Check sheet for the modelled part. Datum: model origin and axes. Units: mm. Face numbers are marked on the shaded views. A direction names the side the tool comes from. Round coordinates to 2 decimals unless told otherwise and drop trailing zeros. Loops run counter-clockwise (first coordinate to the right, second up) from the corner with the lowest first, then second, coordinate; pieces in that order, holes last. Notation, with made-up numbers: (-2.5, 48.25) - (42.5, 48.25) arc R19 cw to (42.5, 82.25) - close; hole circle Ø10 at (-5, 74.5). An arc over 180 degrees is marked (long way). Return JSON: item names as keys, results as strings.
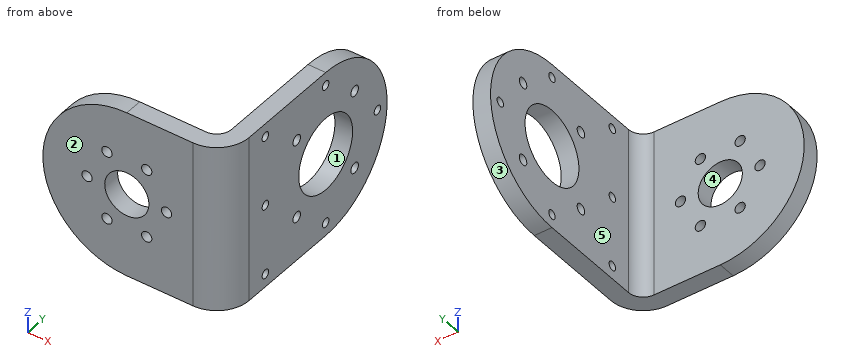
from build123d import *

# Parameters (mm, degrees)
EXTRUDE_1_DEPTH     = 6
EXTRUDE_2_DEPTH     = 6
SKETCH_4_R          = 1.75
CUT_EXTRUDE_1_DEPTH = 16
SKETCH_6_R          = 1.75
CUT_EXTRUDE_2_DEPTH = 16
FILLET_1_R          = 5
FILLET_2_R          = 11
SKETCH_7_R          = 1.5
SKETCH_7_R_2        = 12.5
CUT_EXTRUDE_3_DEPTH = 10
SKETCH_8_R          = 7.5
CUT_EXTRUDE_4_DEPTH = 10


with BuildPart() as part:
    # 草图1 → 凸台-拉伸1 (new body)
    with BuildSketch(Plane(origin=(0, 0, 0), x_dir=(1, 0, 0), z_dir=(0, 1, 0))):
        with BuildLine():
            ThreePointArc((0, 28.5), (-28.5, 0), (0, -28.5))
            Line((0, -28.5), (33.5, -28.5))
            Line((33.5, -28.5), (33.5, 28.5))
            Line((33.5, 28.5), (0, 28.5))
        make_face()
    extrude(amount=EXTRUDE_1_DEPTH)

    # 草图3 → 凸台-拉伸2 (add)
    with BuildSketch(Plane(origin=(33.5, 0, 0), x_dir=(0, 0, -1), z_dir=(1, 0, 0))):
        with BuildLine():
            Line((-28.5, 46.5), (-28.5, 6))
            Line((-28.5, 6), (28.5, 6))
            Line((28.5, 6), (28.5, 46.5))
            ThreePointArc((28.5, 46.5), (0, 75), (-28.5, 46.5))
        make_face()
    extrude(amount=-EXTRUDE_2_DEPTH)

    # 草图4 → 切除-拉伸1 (cut)
    with BuildSketch(Plane(origin=(0, 6, 0), x_dir=(1, 0, 0), z_dir=(0, 1, 0))):
        with Locations(Location((-13.5, 0, 0), (0, 0, 270))):
            Circle(SKETCH_4_R)
        with Locations(Location((-6.75, 11.691342951, 0), (0, 0, 270))):
            Circle(SKETCH_4_R)
        with Locations(Location((6.75, 11.691342951, 0), (0, 0, 270))):
            Circle(SKETCH_4_R)
        with Locations(Location((13.5, 0, 0), (0, 0, 270))):
            Circle(SKETCH_4_R)
        with Locations(Location((6.75, -11.691342951, 0), (0, 0, 270))):
            Circle(SKETCH_4_R)
        with Locations(Location((-6.75, -11.691342951, 0), (0, 0, 270))):
            Circle(SKETCH_4_R)
    extrude(amount=-CUT_EXTRUDE_1_DEPTH, mode=Mode.SUBTRACT)

    # 草图6 → 切除-拉伸2 (cut)
    with BuildSketch(Plane(origin=(33.5, 0, 0), x_dir=(0, 0, -1), z_dir=(1, 0, 0))):
        with Locations((-13.435028843, 59.935028843)):
            Circle(SKETCH_6_R)
        with Locations((13.435028843, 59.935028843)):
            Circle(SKETCH_6_R)
        with Locations((13.435028843, 33.064971157)):
            Circle(SKETCH_6_R)
        with Locations((-13.435028843, 33.064971157)):
            Circle(SKETCH_6_R)
    extrude(amount=-CUT_EXTRUDE_2_DEPTH, mode=Mode.SUBTRACT)

    # 圆角1
    fillet_1_edges = [part.edges().sort_by_distance(p)[0] for p in [
        (27.5, 6, 0),
    ]]
    fillet(fillet_1_edges, radius=FILLET_1_R)

    # 圆角2
    fillet_2_edges = [part.edges().sort_by_distance(p)[0] for p in [
        (33.5, 0, 0),
    ]]
    fillet(fillet_2_edges, radius=FILLET_2_R)

    # 草图7 → 切除-拉伸3 (cut)
    with BuildSketch(Plane(origin=(33.5, 0, 0), x_dir=(0, 0, -1), z_dir=(1, 0, 0))):
        with Locations((0, 70.5)):
            Circle(SKETCH_7_R)
        with Locations((-24, 46.5)):
            Circle(SKETCH_7_R)
        with Locations((24, 46.5)):
            Circle(SKETCH_7_R)
        with Locations((-24, 18.5)):
            Circle(SKETCH_7_R)
        with Locations((24, 18.5)):
            Circle(SKETCH_7_R)
        with Locations((0, 18.5)):
            Circle(SKETCH_7_R)
        with Locations((0, 46.5)):
            Circle(SKETCH_7_R_2)
    extrude(amount=-CUT_EXTRUDE_3_DEPTH, mode=Mode.SUBTRACT)

    # 草图8 → 切除-拉伸4 (cut)
    with BuildSketch(Plane(origin=(0, 6, 0), x_dir=(1, 0, 0), z_dir=(0, 1, 0))):
        with Locations(Location((0, 0, 0), (0, 0, 270))):
            Circle(SKETCH_8_R)
    extrude(amount=-CUT_EXTRUDE_4_DEPTH, mode=Mode.SUBTRACT)


solid = part.part
Q1. Sectioned sample at C-C (y = 52). Enter the section's corners in (x, z), plus the area to 3 significant figures.
Answer key:
{"outline": "(27.5, -27.96) - (33.5, -27.96) - (33.5, -11.22) - (27.5, -11.22) - close; (27.5, 11.22) - (33.5, 11.22) - (33.5, 27.96) - (27.5, 27.96) - close", "area": "201 mm²"}
Q2. Tool access check on the marked faces 4 and 5. Record the directions out of +Z, -Z, +X, -X, +Y, -Y that give a thin tool (end or side, any length) a straight path to the whole face; none if there is none.
Answer key:
{"face 4": "+Y, -Y", "face 5": "+Z, -Z, -X, +Y"}
Q3. Depth check by flat-ended pin: P1, Ø3, axis at y = 33.06, z = 13.44, coming from the -X side; P2, Ø12, axis at x = -3.5, z = -0.5, coming from the +Y side; P3, Ø1, axis at x = 24, z = 5.5, coming from the -Y side; P4, Ø2, axis at y = 31.5, z = 15.5, coming from the -X side. Enter the tip coordinate at first touch or a pass-through.
Answer key:
{"P1": "passes through", "P2": "stops at y = 6", "P3": "stops at y = 0.05", "P4": "stops at x = 27.5"}
Q4. Sectioned sample at A-A (y = 18.5). Enter the section's corners in (x, z).
Answer key:
{"outline": "(27.5, -28.5) - (33.5, -28.5) - (33.5, -25.5) - (27.5, -25.5) - close; (27.5, -22.5) - (33.5, -22.5) - (33.5, -1.5) - (27.5, -1.5) - close; (27.5, 1.5) - (33.5, 1.5) - (33.5, 22.5) - (27.5, 22.5) - close; (27.5, 25.5) - (33.5, 25.5) - (33.5, 28.5) - (27.5, 28.5) - close"}
Q5. Scan lines: probe 1 along Y at (x, z) = (29, -23); probe 2 along Z at (x, y) = (28, 18); probe 3 along Y at (x, z) = (29, 24). Record each from-to range of solid material in increasing order. Write a range as [from, to].
Answer key:
{"probe 1": "y = [2.13, 17.38], [19.62, 45.38], [47.62, 63.33]", "probe 2": "z = [-28.5, -25.41], [-22.59, -1.41], [1.41, 22.59], [25.41, 28.5]", "probe 3": "y = [2.13, 17], [20, 45], [48, 61.87]"}
Q6. Draft check along Y on the marked faces 1, 2 and 3. Enter one of: released by +Y, released by -Y, zero draft, split by the parting line, or undercut.
Answer key:
{"face 1": "undercut", "face 2": "released by -Y", "face 3": "released by +Y"}
Q7. Sectioned sample at D-D (z = -24). Enter the section's corners in (x, y), plus the area to 3 significant figures.
Answer key:
{"outline": "(-15.37, 0) - (22.5, 0) arc R11 ccw to (33.5, 11) - (33.5, 17) - (27.5, 17) - (27.5, 11) arc R5 cw to (22.5, 6) - (-15.37, 6) - close; (27.5, 20) - (33.5, 20) - (33.5, 45) - (27.5, 45) - close; (27.5, 48) - (33.5, 48) - (33.5, 61.87) - (27.5, 61.87) - close", "area": "572 mm²"}
Q8. Sectioned sample at B-B (z = 0). State how many separate pieces and enclosed holes the cut face has, plus the area to 3 significant figures.
Answer key:
{"separate pieces": "7", "enclosed holes": "0", "area": "447 mm²"}
